```python
from build123d import *

# Parameters (mm, degrees)
SALIENTE_EXTRUIR1_DEPTH      = 20
SALIENTE_EXTRUIR2_DEPTH      = 20
SALIENTE_EXTRUIR2_DEPTH_BACK = 60
CROQUIS2_W                   = 19.396492872
CROQUIS2_H                   = 26
CORTAR_EXTRUIR1_DEPTH        = 18
CORTAR_EXTRUIR1_DEPTH_BACK   = 18
CORTAR_EXTRUIR1_START        = -20
CROQUIS4_W                   = 66
CROQUIS4_H                   = 36
CORTAR_EXTRUIR2_DEPTH        = 9
CORTAR_EXTRUIR2_DEPTH_BACK   = 9
CORTAR_EXTRUIR2_START        = -13
CROQUIS6_W                   = 11.396492872
CROQUIS6_H                   = 72


with BuildPart() as part:
    # Croquis1 → Saliente-Extruir1 (new, symmetric)
    with BuildSketch(Plane.XY):
        Polygon((65.424276511, 73.988341167), (80.72172581, 47.492381754), (102.372360904, 59.992381754), (85.074911605, 89.952442782), (29.226887967, 57.7085713), (-40.773112033, 57.7085713), (-40.773112033, 17.7085713), (29.226887967, 17.7085713), (29.226887967, 53.089769147), align=None)
    extrude(amount=SALIENTE_EXTRUIR1_DEPTH, both=True)

    # Croquis2 → Saliente-Extruir2 (add, two sides: drawn at the far end of the back side and taken through both)
    with BuildSketch(Plane(origin=(0, 57.7085713, 0), x_dir=(1, 0, 0), z_dir=(0, 1, 0)).offset(-SALIENTE_EXTRUIR2_DEPTH_BACK)):
        with Locations((-23.273112033, 0)):
            Rectangle(CROQUIS2_W, CROQUIS2_H)
    extrude(amount=SALIENTE_EXTRUIR2_DEPTH + SALIENTE_EXTRUIR2_DEPTH_BACK)

    # Croquis4 → Cortar-Extruir1 (cut, two sides: drawn at the far end of the back side and taken through both)
    with BuildSketch(Plane.XY.offset(20).offset(CORTAR_EXTRUIR1_START - CORTAR_EXTRUIR1_DEPTH_BACK)):
        with Locations((-5.773112033, 37.7085713)):
            Rectangle(CROQUIS4_W, CROQUIS4_H)
    extrude(amount=CORTAR_EXTRUIR1_DEPTH + CORTAR_EXTRUIR1_DEPTH_BACK, mode=Mode.SUBTRACT)

    # Croquis6 → Cortar-Extruir2 (cut, two sides: drawn at the far end of the back side and taken through both)
    with BuildSketch(Plane.XY.offset(13).offset(CORTAR_EXTRUIR2_START - CORTAR_EXTRUIR2_DEPTH_BACK)):
        with Locations((-23.273112033, 37.7085713)):
            Rectangle(CROQUIS6_W, CROQUIS6_H)
    extrude(amount=CORTAR_EXTRUIR2_DEPTH + CORTAR_EXTRUIR2_DEPTH_BACK, mode=Mode.SUBTRACT)


solid = part.part
```
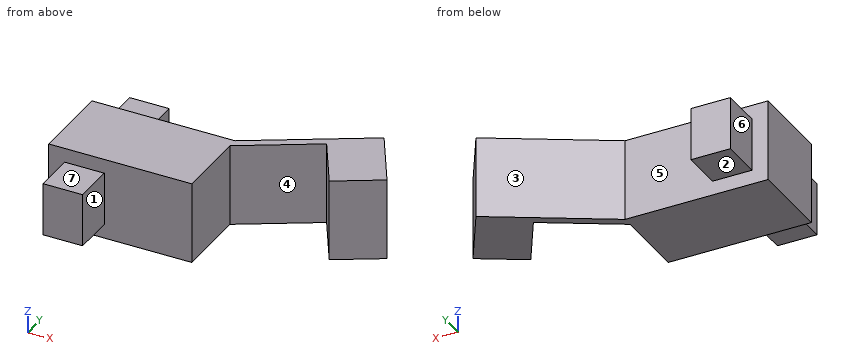
Here's how the part is built. I have some questions about the finished solid (model axes, mm). Face numbers are marked on the shaded views. A direction names the side the tool comes from. Round coordinates to 2 decimals unless told otherwise and drop trailing zeros. Loops run counter-clockwise (first coordinate to the right, second up) from the corner with the lowest first, then second, coordinate; pieces in that order, holes last. Notation, with made-up numbers: (-38, 69.5) -> (-25, 69.5) arc R20 ccw to (-25, 98.5) -> close; hole circle Ø9 at (40, 37). An arc over 180 degrees is marked (long way). Answer as CSV lines item,"result".
1. If we section it at B-B on z = 15.5: Please give me the cut outline in (x, y).
Final values:
outline,"(-40.77, 17.71) -> (29.23, 17.71) -> (29.23, 53.09) -> (65.42, 73.99) -> (80.72, 47.49) -> (102.37, 59.99) -> (85.07, 89.95) -> (29.23, 57.71) -> (-40.77, 57.71) -> close; hole (-38.77, 19.71) -> (27.23, 19.71) -> (27.23, 55.71) -> (-38.77, 55.71) -> close"
2. If we section it at C-C on y = 67: Please give me the cut outline in (x, z), plus the area to 3 significant figures.
Final values:
outline,"(-32.97, -13) -> (-13.57, -13) -> (-13.57, 13) -> (-32.97, 13) -> close; (45.32, -20) -> (53.32, -20) -> (53.32, 20) -> (45.32, 20) -> close; (69.46, -20) -> (98.33, -20) -> (98.33, 20) -> (69.46, 20) -> close; hole (-28.97, -9) -> (-17.57, -9) -> (-17.57, 9) -> (-28.97, 9) -> close"
area,"1,770 mm^2"
3. If we section it at A-A on x = -25.5: Please give me the cut outline in (y, z), plus the area to 3 significant figures.
Final values:
outline,"(-2.29, -13) -> (17.71, -13) -> (17.71, -20) -> (57.71, -20) -> (57.71, -13) -> (77.71, -13) -> (77.71, 13) -> (57.71, 13) -> (57.71, 20) -> (17.71, 20) -> (17.71, 13) -> (-2.29, 13) -> close; hole (1.71, -9) -> (19.71, -9) -> (19.71, -18) -> (55.71, -18) -> (55.71, -9) -> (73.71, -9) -> (73.71, 9) -> (55.71, 9) -> (55.71, 18) -> (19.71, 18) -> (19.71, 9) -> (1.71, 9) -> close"
area,"696 mm^2"
4. If we section it at D-D on y = 32: Please give me the cut outline in (x, z).
Final values:
outline,"(-40.77, -20) -> (29.23, -20) -> (29.23, 20) -> (-40.77, 20) -> close; hole (-38.77, -18) -> (27.23, -18) -> (27.23, 18) -> (-38.77, 18) -> close"
5. For pin 1 (2 mm diameter, centred on x = 20.5, z = 11, fed in from +Y); pin 2 (12.5 mm diameter, centred on x = -21.5, y = 65.5, fed in from -Z); pin 3 (4 mm diameter, centred on x = 26.5, z = -8, fed in from -Y), each with a flat end and sliding along its axis, tell me the tip position at first contact or that it passes through.
Final values:
pin 1,"stops at y = 57.71"
pin 2,"stops at z = -13"
pin 3,"stops at y = 17.71"
6. Thinking about a two-plate mould opening in X: for the marked faces 5, 6 and 7, which applies, released by +X, released by -X, zero draft, split by the parting line, or undercut?
Final values:
face 5,"undercut"
face 6,"released by -X"
face 7,"zero draft"
7. Which directions (+Z, -Z, +X, -X, +Y, -Y) give clear straight access to the entire face, cutting with the end or side of a thin tool? Please do the marked faces 1, 2, 3 and 4.
Final values:
face 1,"+Z, -Z, +X, -Y"
face 2,"-Z, -X, +Y"
face 3,"+Z, -Z, +Y"
face 4,"+Z, -Z, -Y"
8. If I drill on L1, parallel to X at y = 18, z = -8.5; L2, parallel to Y at x = 6.5, z = 9.5; L3, parallel to X at y = 65.5, z = -2, over which ranges is the centre line in solid material (lowest first)?
Final values:
L1,"x = -40.77 to -28.97, -17.57 to 29.23"
L2,"y = 17.71 to 19.71, 55.71 to 57.71"
L3,"x = -32.97 to -28.97, -17.57 to -13.57, 42.72 to 50.72, 70.33 to 99.19"
